Check sheet for the modelled part. Datum: model origin and axes. Units: mm. Coordinates: 2 decimals unless noted, no trailing zeros. Loops run counter-clockwise (first coordinate to the right, second up) from the corner with the lowest first, then second, coordinate; pieces in that order, holes last. Notation, with made-up numbers: M 49,52 L 87,52 A17 ccw 87,83 Z; hole C -3.5,71.5 d6. An arc over 180 degrees is marked long. Return JSON: item names as keys, results as strings.
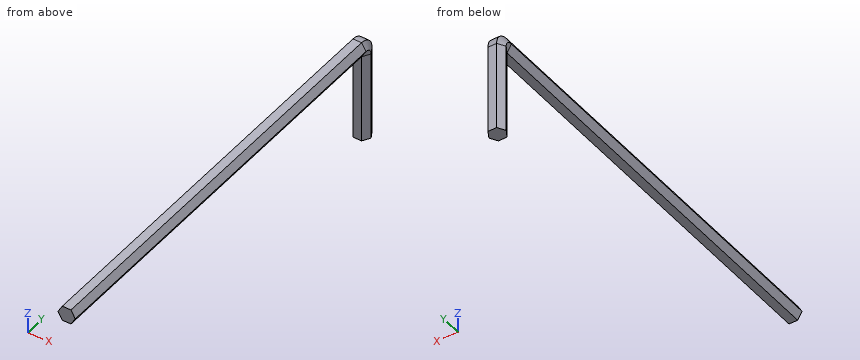
from build123d import *

# Parameters (mm, degrees)
F1_DEPTH = 15
F3_ANGLE = 90
F5_DEPTH = 70


with BuildPart() as f1:
    # F0 (on Top) → F1 (new body)
    with BuildSketch(Plane.XY):
        Polygon((0.7031400781, -1.2605266217), (1.4432181155, -0.0213261408), (0.7400780375, 1.2392004809), (-0.7031400781, 1.2605266217), (-1.4432181155, 0.0213261408), (-0.7400780375, -1.2392004809), align=None)
    extrude(amount=F1_DEPTH)

    # F2 (on face) → F3 (revolve)
    with BuildSketch(Plane.XY.offset(15)):
        Polygon((-1.4432181155, 0.0213261408), (-0.7400780375, -1.2392004809), (0.7031400781, -1.2605266217), (1.4432181155, -0.0213261408), (0.7400780375, 1.2392004809), (-0.7031400781, 1.2605266217), align=None)
    revolve(axis=Axis((-0.0184689797, -1.2498635513, 15), (0.999890841, -0.0147751838, 0)), revolution_arc=F3_ANGLE)

    # F4 (on face) → F5 (join)
    with BuildSketch(Plane(origin=(-0.0184689797, -1.2498635513, 0), x_dir=(0.999890841, -0.0147751838, 0), z_dir=(-0.0147751838, -0.999890841, 0))):
        Polygon((-0.7216878365, 15), (0.7216878365, 15), (1.443375673, 16.25), (0.7216878365, 17.5), (-0.7216878365, 17.5), (-1.443375673, 16.25), align=None)
    extrude(amount=F5_DEPTH)


solid = f1.part
1) Section check B-B on y = -4.5. Record the cut outline in (x, z).
Answers:
{"outline": "M -1.51,16.25 L -0.79,15 L 0.66,15 L 1.38,16.25 L 0.66,17.5 L -0.79,17.5 Z"}
2) Scan lines: line 1 along Y through (x, z) = (-0.6, 7.25); line 2 along Z through (x, y) = (-0.45, -15); line 3 along Y through (x, z) = (0.2, 11.75). Record each from-to range of solid material in increasing order. Write a range as [from, to].
Answers:
{"line 1": "[-1.24, 1.26]", "line 2": "[15, 17.5]", "line 3": "[-1.25, 1.25]"}
3) Section check A-A on z = 6.25. Record the cut outline in (x, y), then the cut area to 3 significant figures.
Answers:
{"outline": "M -1.44,0.02 L -0.74,-1.24 L 0.7,-1.26 L 1.44,-0.02 L 0.74,1.24 L -0.7,1.26 Z", "area": "5.41 mm²"}
4) Go/stop test with flat-tipped pins: pin 1 Ø6 at (y, z) = (-30.5, 13) entering from +X; pin 2 Ø2 at (y, z) = (-55, 14.5) entering from -X. Record where each tip stops, or that it passes through.
Answers:
{"pin 1": "x = 0.85", "pin 2": "x = -1.82"}
